Geometry: see drawing. Coordinates: mm, zero at the bounding-box minimum. A direction names the side the tool comes from. Give positions to 0.01 mm unless a question says otherwise; leave off trailing zeros. Use CSV: the item, a comma, the result in double quotes. Start each with the question number.
1) Set-up query: the marked faces 1, 2 and 3. Return all of +Z, -Z, +X, -X, +Y, -Y with unobstructed straight access to the full face (end or side cutting, diameter ignored); none if empty.
2) Contact query for flat-ended pins moving along their axis: P1, Ø6.5, axis at x = 42.075, y = 13.725, coming from the +Z side (1 decimal); P2, Ø4, axis at y = 37.5, z = 33, coming from the -X side; P3, Ø5, axis at x = 15, y = 37.5, coming from the +Z side. Output: stop coordinate, or through.
3) Draft query along Y for the marked faces 4, 5 and 6. Return one class per face: pulls with the +Y half, pulls with the -Y half, needs draft (parallel to the pull), parting line crosses it, or undercut.
4) Material intervals for line 1 (Z direction, x = 54, y = 18.5) (1 decimal); line 2 (X direction, y = 36, z = 14); line 3 (Z direction, x = 9, y = 27) (1 decimal), sorted ascending. Write a range as [from, to].
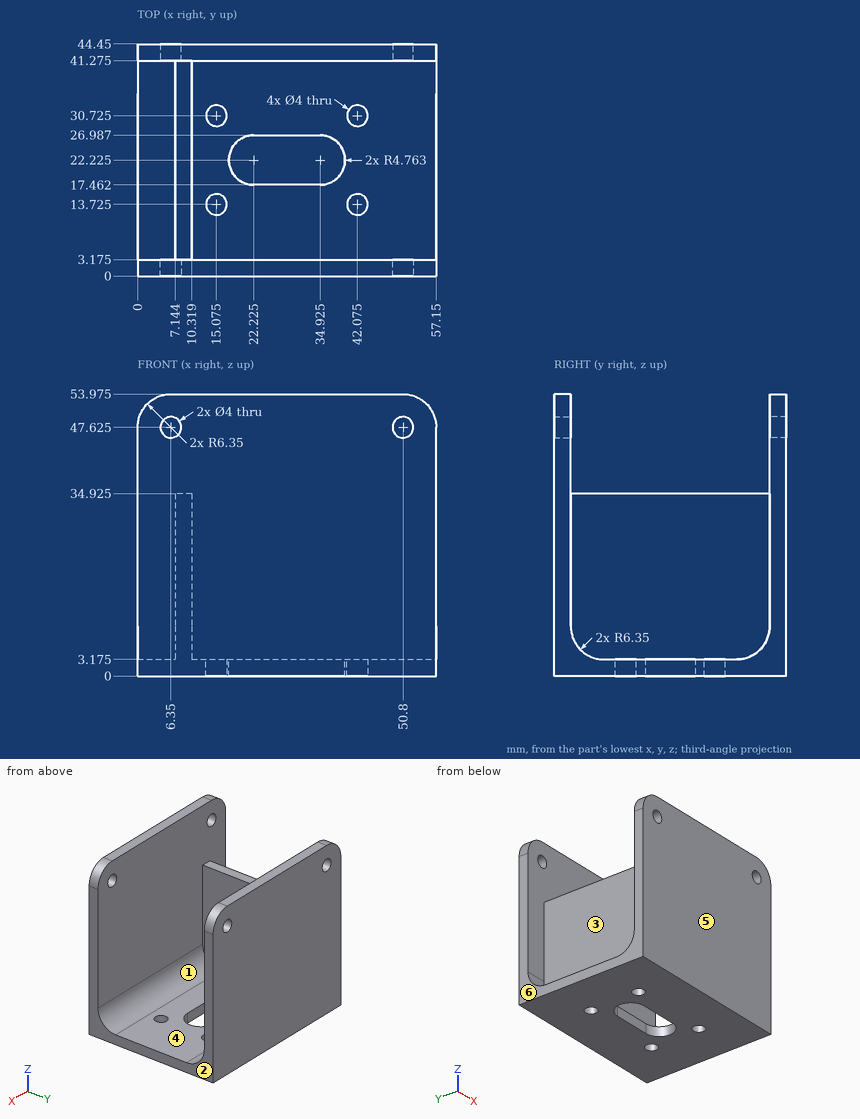
Answers follow:
1,face 1,"+Z, +X"
1,face 2,"+Z, -Z, +X, +Y, -Y"
1,face 3,"+Z, -X"
2,P1,"stops at z = 3.2"
2,P2,"stops at x = 7.14"
2,P3,"stops at z = 5.71"
3,face 4,"undercut"
3,face 5,"pulls with the -Y half"
3,face 6,"needs draft"
4,line 1,"z = [0, 3.2]"
4,line 2,"x = [7.14, 10.32]"
4,line 3,"z = [0, 34.9]"
